Read the model definition and answer for the solid it produces. Units are mm, in the model's axes. Face numbers are marked on the shaded views. Give positions to 0.01 mm unless a question says otherwise; leave off trailing zeros. Loops run counter-clockwise (first coordinate to the right, second up) from the corner with the lowest first, then second, coordinate; pieces in that order, holes last. Notation, with made-up numbers: (-21, 22) -> (30, 22) arc R27 ccw to (30, 54) -> close; hole circle Ø5 at (11, 17.5). An arc over 180 degrees is marked (long way). One line per item, written item: value. Start each with the question number.
from build123d import *

# Parameters (mm, degrees)
SKETCH1_W           = 127
SKETCH1_H           = 190.5
BOSS_EXTRUDE1_DEPTH = 63.5
SKETCH4_W           = 127
SKETCH4_H           = 71.842048968
CUT_EXTRUDE1_DEPTH  = 63.5
SKETCH5_R           = 12.7
CUT_EXTRUDE2_DEPTH  = 137.16
BOSS_EXTRUDE2_DEPTH = 127


with BuildPart() as part:
    # Sketch1 → Boss-Extrude1 (new body)
    with BuildSketch(Plane.XY):
        Rectangle(SKETCH1_W, SKETCH1_H)
    extrude(amount=BOSS_EXTRUDE1_DEPTH)

    # Sketch4 → Cut-Extrude1 (cut)
    with BuildSketch(Plane(origin=(0, -22.225, -22.225), x_dir=(1, 0, 0), z_dir=(0, 0.7071067811865477, 0.7071067811865475))):
        with Locations((0, -67.351920908)):
            Rectangle(SKETCH4_W, SKETCH4_H)
    cut_extrude1 = extrude(amount=-CUT_EXTRUDE1_DEPTH, mode=Mode.SUBTRACT)

    # Sketch5 → Cut-Extrude2 (cut)
    with BuildSketch(Plane(origin=(63.5, 0, 0), x_dir=(0, 0, -1), z_dir=(1, 0, 0))):
        with Locations((-25.4, 0)):
            Circle(SKETCH5_R)
    extrude(amount=-CUT_EXTRUDE2_DEPTH, mode=Mode.SUBTRACT)

    # Mirror1: Cut-Extrude1 across plane
    add(cut_extrude1.mirror(Plane.ZX), mode=Mode.SUBTRACT)

    # Sketch7 → Boss-Extrude2 (add)
    with BuildSketch(Plane(origin=(63.5, 0, 0), x_dir=(0, 0, -1), z_dir=(1, 0, 0))):
        Polygon((-63.5, 95.25), (-88.9, 95.25), (-63.5, 0), align=None)
    extrude(amount=-BOSS_EXTRUDE2_DEPTH)


solid = part.part
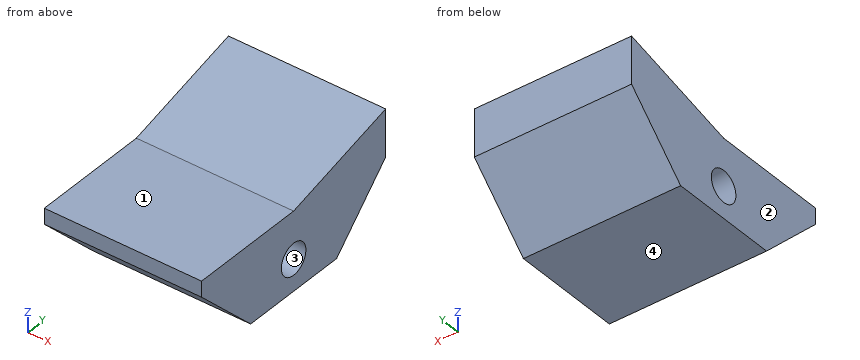
Item 1: Section A-A, the plane z = 25.4 is taken. Determine the outline of the cut face in (x, y).
Item 2: Section C-C, the plane z = 6 is taken. Determine the outline of the cut face in (x, y), plus the area to 3 significant figures.
Item 3: Flat-ended cylindrical pins translate along their axes: pin 1 (12 mm diameter, centred on x = -16.5, z = 9.5, fed in from -Y); pin 2 (5 mm diameter, centred on x = -12, z = 28.5, fed in from +Y). Find the tip coordinate at first contact, or state that the pin passes through.
Item 4: Consider L1, parallel to Y at x = -8, z = 25; L2, parallel to Y at x = -7, z = 15.5; L3, parallel to Z at x = -14.5, y = -13. Determine where each line is inside the solid, lowest interval first. Write a range as [from, to].
Item 5: Section B-B, the plane x = 35.5 is taken. Determine the outline of the cut face in (y, z), plus the area to 3 significant figures.
Item 6: Section D-D, the plane y = 37 is taken. Determine the outline of the cut face in (x, z), plus the area to 3 significant figures.
Item 7: Determine the mould class of the marked faces 1, 2, 3 and 4 for opening direction Z: pulls with the +Z half, pulls with the -Z half, needs draft (parallel to the pull), parting line crosses it, or undercut.
Computed values:
1. outline: (-63.5, -69.85) -> (63.5, -69.85) -> (63.5, -12.7) -> (-63.5, -12.7) -> close; (-63.5, 12.7) -> (63.5, 12.7) -> (63.5, 69.85) -> (-63.5, 69.85) -> close
2. outline: (-63.5, -50.45) -> (63.5, -50.45) -> (63.5, 50.45) -> (-63.5, 50.45) -> close
2. area: 12,800 mm²
3. pin 1: y = -59.95
3. pin 2: y = 75.45
4. L1: [-69.45, -12.69], [12.69, 69.45]
4. L2: [-59.95, -7.95], [7.95, 59.95]
4. L3: [0, 63.5]
5. outline: (-95.25, 50.8) -> (-44.45, 0) -> (44.45, 0) -> (95.25, 50.8) -> (95.25, 88.9) -> (0, 63.5) -> (-95.25, 63.5) -> close; hole circle Ø25.4 at (0, 25.4)
5. area: 10,200 mm²
6. outline: (-63.5, 0) -> (63.5, 0) -> (63.5, 73.37) -> (-63.5, 73.37) -> close
6. area: 9,320 mm²
7. face 1: pulls with the +Z half
7. face 2: needs draft
7. face 3: undercut
7. face 4: pulls with the -Z half
